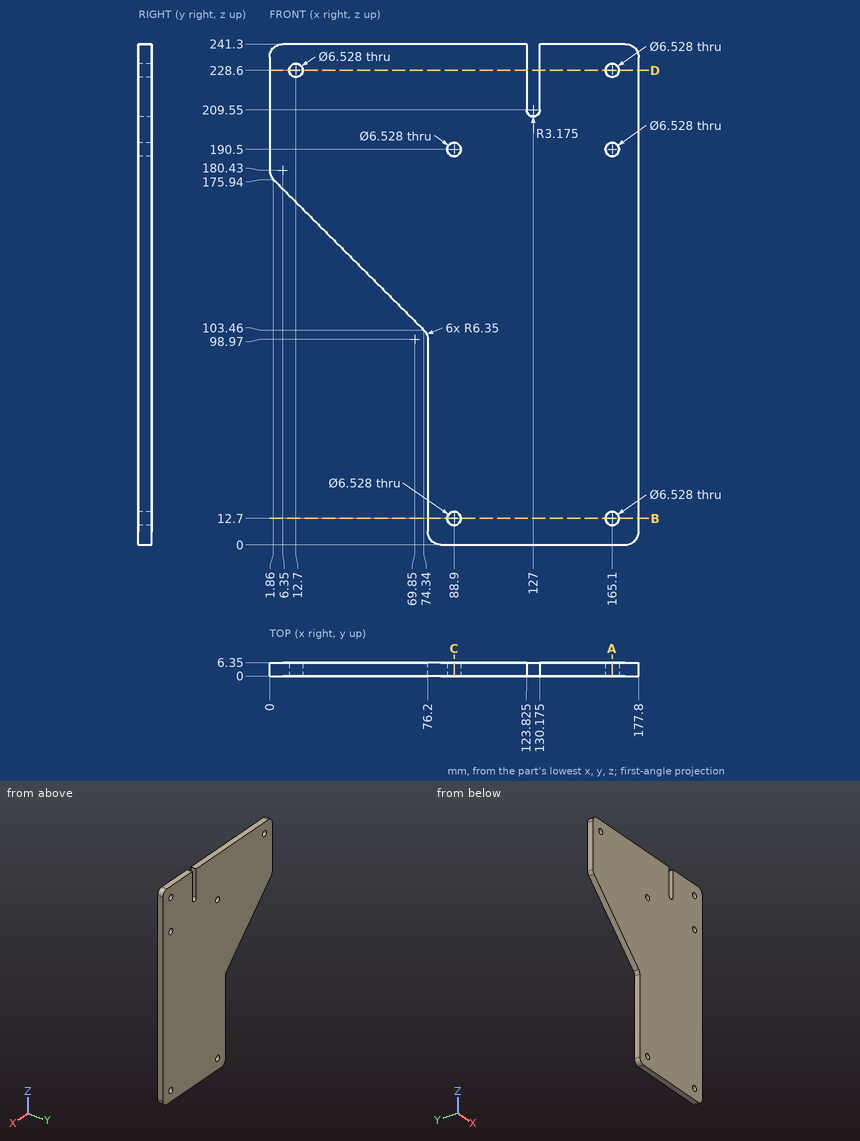
Source: three-view drawing plus pictorial views. Frame: mm from the lowest corner of the part. Round coordinates to 2 decimals unless told otherwise and drop trailing zeros. Loops run counter-clockwise (first coordinate to the right, second up) from the corner with the lowest first, then second, coordinate; pieces in that order, holes last. Notation, with made-up numbers: (-32.75, 55) -> (0.25, 55) arc R23 cw to (0.25, 67) -> close; hole circle Ø10 at (-35.5, 61.5). An arc over 180 degrees is marked (long way). Use one line per item in the form item = value.
Item 1: Cut plane D-D on z = 228.6. Give the number of separate pieces and of enclosed holes in the cut face, then the cut area to 3 significant figures.
Evaluation:
separate_pieces = 4
enclosed_holes = 0
area = 1,010 mm2
Item 2: Cut plane C-C on x = 88.9. Output: boundary loops of the cut face in (y, z).
Evaluation:
outline = (0, 0) -> (6.35, 0) -> (6.35, 9.44) -> (0, 9.44) -> close; (0, 15.96) -> (6.35, 15.96) -> (6.35, 187.24) -> (0, 187.24) -> close; (0, 193.76) -> (6.35, 193.76) -> (6.35, 241.3) -> (0, 241.3) -> close
Item 3: Material intervals for probe 1 along X at (y, z) = (2.25, 190.5); probe 2 along X at (y, z) = (4, 228.6) (1 decimal); probe 3 along X at (y, z) = (4, 12.7), sorted ascending.
Evaluation:
probe_1 = 0 to 85.64, 92.16 to 161.84, 168.36 to 177.8
probe_2 = 0 to 9.4, 16 to 123.8, 130.2 to 161.8, 168.4 to 177.8
probe_3 = 76.2 to 85.64, 92.16 to 161.84, 168.36 to 177.8
Item 4: Cut plane A-A on x = 165.1. Output: boundary loops of the cut face in (y, z), then the cut area to 3 significant figures.
Evaluation:
outline = (0, 0) -> (6.35, 0) -> (6.35, 9.44) -> (0, 9.44) -> close; (0, 15.96) -> (6.35, 15.96) -> (6.35, 187.24) -> (0, 187.24) -> close; (0, 193.76) -> (6.35, 193.76) -> (6.35, 225.34) -> (0, 225.34) -> close; (0, 231.86) -> (6.35, 231.86) -> (6.35, 241.3) -> (0, 241.3) -> close
area = 1,410 mm2
Item 5: Contact query for flat-ended pins moving along their axis: pin 1 Ø4 at (x, z) = (12.7, 228.6) entering from +Y; pin 2 Ø1 at (x, y) = (32.5, 3) entering from -Z. Output: stop coordinate, or through.
Evaluation:
pin_1 = through
pin_2 = 144.8
Item 6: Cut plane B-B on z = 12.7. Output: boundary loops of the cut face in (x, y), then the cut area to 3 significant figures.
Evaluation:
outline = (76.2, 0) -> (85.64, 0) -> (85.64, 6.35) -> (76.2, 6.35) -> close; (92.16, 0) -> (161.84, 0) -> (161.84, 6.35) -> (92.16, 6.35) -> close; (168.36, 0) -> (177.8, 0) -> (177.8, 6.35) -> (168.36, 6.35) -> close
area = 562 mm2
